Here's how the part is built. I have some questions about the finished solid (model axes, mm). A direction names the side the tool comes from. Coordinates: 2 decimals unless noted, no trailing zeros. Use CSV: the item, a comma, the result in double quotes. Start each with the question number.
```python
from build123d import *

# Parameters (mm, degrees)
ARM_DEPTH            = 2.54
LIGHTING_HOLES_REACH = 407.324
SKETCH3_R            = 10.563906398
SKETCH3_R_2          = 12.998589321
SKETCH3_R_3          = 14.959386689
SKETCH3_R_4          = 18.989420404
SKETCH3_R_5          = 20.414251761
SKETCH3_R_6          = 9.810598177
PIVOT_HOLES_REACH    = 407.324
SKETCH4_R            = 6.35
SKETCH5_R            = 2.54
EDGE_HOLES_DEPTH     = 2.54


with BuildPart() as part:
    # Sketch2 → Arm (new body)
    with BuildSketch(Plane(origin=(0, 0, 0), x_dir=(1, 0, 0), z_dir=(0, 1, 0))):
        with BuildLine():
            Line((-196.324159543, 163.36805283), (-239.26276826, 99.105883584))
            Line((-239.26276826, 99.105883584), (-258.976154185, 0))
            Line((-258.976154185, 0), (-239.26276826, -99.105883584))
            Line((-239.26276826, -99.105883584), (-183.12379479, -183.12379479))
            Line((-183.12379479, -183.12379479), (-110.768588535, -231.469997952))
            ThreePointArc((-110.768588535, -231.469997952), (-104.473118761, -249.064657285), (-119.482679559, -260.19650625))
            Line((-119.482679559, -260.19650625), (-231.805977786, -260.19650625))
            ThreePointArc((-231.805977786, -260.19650625), (-238.01719804, -258.573994365), (-242.641366534, -254.121032698))
            Line((-242.641366534, -254.121032698), (-263.949339301, -219.268704737))
            Line((-263.949339301, -219.268704737), (-305.536674142, -121.363782023))
            Line((-305.536674142, -121.363782023), (-310.771385022, 0))
            Line((-310.771385022, 0), (-287.766347466, 115.654133822))
            ThreePointArc((-287.766347466, 115.654133822), (-286.898137133, 118.373962558), (-285.444305631, 120.831121792))
            Line((-285.444305631, 120.831121792), (-238.69541851, 182.721728369))
            ThreePointArc((-238.69541851, 182.721728369), (-234.221705245, 186.435995307), (-228.561487284, 187.76709331))
            Line((-228.561487284, 187.76709331), (-209.365718386, 187.76709331))
            ThreePointArc((-209.365718386, 187.76709331), (-195.532827931, 179.475977845), (-196.324159543, 163.36805283))
        make_face()
    extrude(amount=ARM_DEPTH)

    # Sketch3 → Lighting Holes (cut, up to next)
    with BuildSketch(Plane(origin=(0, 2.54, 0), x_dir=(1, 0, 0), z_dir=(0, 1, 0)), mode=Mode.PRIVATE) as lighting_holes_sk1:
        with Locations(Location((-262.564493281, 112.317651632, 0), (0, 0, 270))):
            Circle(SKETCH3_R)
    lighting_holes_tool1 = extrude(lighting_holes_sk1.sketch, amount=-LIGHTING_HOLES_REACH, mode=Mode.PRIVATE) & part.part
    # Sketch3 → Lighting Holes (cut, up to next)
    with BuildSketch(Plane(origin=(0, 2.54, 0), x_dir=(1, 0, 0), z_dir=(0, 1, 0)), mode=Mode.PRIVATE) as lighting_holes_sk2:
        with Locations(Location((-273.830034517, 62.17947414, 0), (0, 0, 270))):
            Circle(SKETCH3_R_2)
    lighting_holes_tool2 = extrude(lighting_holes_sk2.sketch, amount=-LIGHTING_HOLES_REACH, mode=Mode.PRIVATE) & part.part
    # Sketch3 → Lighting Holes (cut, up to next)
    with BuildSketch(Plane(origin=(0, 2.54, 0), x_dir=(1, 0, 0), z_dir=(0, 1, 0)), mode=Mode.PRIVATE) as lighting_holes_sk3:
        with Locations(Location((-283.210721504, 0, 0), (0, 0, 270))):
            Circle(SKETCH3_R_3)
    lighting_holes_tool3 = extrude(lighting_holes_sk3.sketch, amount=-LIGHTING_HOLES_REACH, mode=Mode.PRIVATE) & part.part
    # Sketch3 → Lighting Holes (cut, up to next)
    with BuildSketch(Plane(origin=(0, 2.54, 0), x_dir=(1, 0, 0), z_dir=(0, 1, 0)), mode=Mode.PRIVATE) as lighting_holes_sk4:
        with Locations(Location((-275.563082601, -58.328881999, 0), (0, 0, 270))):
            Circle(SKETCH3_R_4)
    lighting_holes_tool4 = extrude(lighting_holes_sk4.sketch, amount=-LIGHTING_HOLES_REACH, mode=Mode.PRIVATE) & part.part
    # Sketch3 → Lighting Holes (cut, up to next)
    with BuildSketch(Plane(origin=(0, 2.54, 0), x_dir=(1, 0, 0), z_dir=(0, 1, 0)), mode=Mode.PRIVATE) as lighting_holes_sk5:
        with Locations(Location((-268.251334815, -119.393093751, 0), (0, 0, 270))):
            Circle(SKETCH3_R_5)
    lighting_holes_tool5 = extrude(lighting_holes_sk5.sketch, amount=-LIGHTING_HOLES_REACH, mode=Mode.PRIVATE) & part.part
    # Sketch3 → Lighting Holes (cut, up to next)
    with BuildSketch(Plane(origin=(0, 2.54, 0), x_dir=(1, 0, 0), z_dir=(0, 1, 0)), mode=Mode.PRIVATE) as lighting_holes_sk6:
        with Locations(Location((-229.533929598, 151.758024286, 0), (0, 0, 270))):
            Circle(SKETCH3_R_6)
    lighting_holes_tool6 = extrude(lighting_holes_sk6.sketch, amount=-LIGHTING_HOLES_REACH, mode=Mode.PRIVATE) & part.part
    add(lighting_holes_tool1.solids().sort_by_distance((-262.564493, 2.54, -112.317652))[0], mode=Mode.SUBTRACT)
    add(lighting_holes_tool2.solids().sort_by_distance((-273.830035, 2.54, -62.179474))[0], mode=Mode.SUBTRACT)
    add(lighting_holes_tool3.solids().sort_by_distance((-283.210722, 2.54, 0))[0], mode=Mode.SUBTRACT)
    add(lighting_holes_tool4.solids().sort_by_distance((-275.563083, 2.54, 58.328882))[0], mode=Mode.SUBTRACT)
    add(lighting_holes_tool5.solids().sort_by_distance((-268.251335, 2.54, 119.393094))[0], mode=Mode.SUBTRACT)
    add(lighting_holes_tool6.solids().sort_by_distance((-229.53393, 2.54, -151.758024))[0], mode=Mode.SUBTRACT)

    # Sketch4 → Pivot Holes (cut, up to next)
    with BuildSketch(Plane(origin=(0, 2.54, 0), x_dir=(1, 0, 0), z_dir=(0, 1, 0)), mode=Mode.PRIVATE) as pivot_holes_sk1:
        with Locations(Location((-119.482679559, -244.511556794, 0), (0, 0, 270))):
            Circle(SKETCH4_R)
    pivot_holes_tool1 = extrude(pivot_holes_sk1.sketch, amount=-PIVOT_HOLES_REACH, mode=Mode.PRIVATE) & part.part
    # Sketch4 → Pivot Holes (cut, up to next)
    with BuildSketch(Plane(origin=(0, 2.54, 0), x_dir=(1, 0, 0), z_dir=(0, 1, 0)), mode=Mode.PRIVATE) as pivot_holes_sk2:
        with Locations(Location((-227.432679559, -244.511556794, 0), (0, 0, 270))):
            Circle(SKETCH4_R)
    pivot_holes_tool2 = extrude(pivot_holes_sk2.sketch, amount=-PIVOT_HOLES_REACH, mode=Mode.PRIVATE) & part.part
    add(pivot_holes_tool1.solids().sort_by_distance((-119.48268, 2.54, 244.511557))[0], mode=Mode.SUBTRACT)
    add(pivot_holes_tool2.solids().sort_by_distance((-227.43268, 2.54, 244.511557))[0], mode=Mode.SUBTRACT)

    # Sketch5 → Edge Holes (cut)
    with BuildSketch(Plane(origin=(0, 2.54, 0), x_dir=(1, 0, 0), z_dir=(0, 1, 0))):
        with Locations(Location((-186.786270686, -186.786270686, 0), (0, 0, 270))):
            Circle(SKETCH5_R)
        with Locations(Location((-200.897754604, -165.666942533, 0), (0, 0, 270))):
            Circle(SKETCH5_R)
        with Locations(Location((-215.009238523, -144.547614381, 0), (0, 0, 270))):
            Circle(SKETCH5_R)
        with Locations(Location((-229.120722442, -123.428286228, 0), (0, 0, 270))):
            Circle(SKETCH5_R)
        with Locations(Location((-244.048023625, -101.088001256, 0), (0, 0, 270))):
            Circle(SKETCH5_R)
        with Locations(Location((-249.003317804, -76.176055134, 0), (0, 0, 270))):
            Circle(SKETCH5_R)
        with Locations(Location((-253.958611984, -51.264109011, 0), (0, 0, 270))):
            Circle(SKETCH5_R)
        with Locations(Location((-258.913906163, -26.352162889, 0), (0, 0, 270))):
            Circle(SKETCH5_R)
        with Locations(Location((-264.155677269, 0, 0), (0, 0, 270))):
            Circle(SKETCH5_R)
        with Locations(Location((-259.200383089, 24.911946122, 0), (0, 0, 270))):
            Circle(SKETCH5_R)
        with Locations(Location((-254.24508891, 49.823892244, 0), (0, 0, 270))):
            Circle(SKETCH5_R)
        with Locations(Location((-249.289794731, 74.735838367, 0), (0, 0, 270))):
            Circle(SKETCH5_R)
        with Locations(Location((-244.048023625, 101.088001256, 0), (0, 0, 270))):
            Circle(SKETCH5_R)
        with Locations(Location((-229.936539706, 122.207329408, 0), (0, 0, 270))):
            Circle(SKETCH5_R)
        with Locations(Location((-215.825055788, 143.326657561, 0), (0, 0, 270))):
            Circle(SKETCH5_R)
        with Locations(Location((-200.548025174, 166.190349614, 0), (0, 0, 270))):
            Circle(SKETCH5_R)
        with Locations(Location((-209.365718386, 182.68709331, 0), (0, 0, 270))):
            Circle(SKETCH5_R)
        with Locations(Location((-249.95111614, 159.392011893, 0), (0, 0, 270))):
            Circle(SKETCH5_R)
        with Locations(Location((-234.64184602, 179.659874346, 0), (0, 0, 270))):
            Circle(SKETCH5_R)
        with Locations(Location((-265.26038626, 139.12414944, 0), (0, 0, 270))):
            Circle(SKETCH5_R)
        with Locations(Location((-282.783958242, 114.663074986, 0), (0, 0, 270))):
            Circle(SKETCH5_R)
        with Locations(Location((-287.739252421, 89.751128864, 0), (0, 0, 270))):
            Circle(SKETCH5_R)
        with Locations(Location((-292.6945466, 64.839182741, 0), (0, 0, 270))):
            Circle(SKETCH5_R)
        with Locations(Location((-297.649840779, 39.927236619, 0), (0, 0, 270))):
            Circle(SKETCH5_R)
        with Locations(Location((-302.605134959, 15.015290497, 0), (0, 0, 270))):
            Circle(SKETCH5_R)
        with Locations(Location((-305.66976845, -0.391662485, 0), (0, 0, 270))):
            Circle(SKETCH5_R)
        with Locations(Location((-304.57522323, -25.768068274, 0), (0, 0, 270))):
            Circle(SKETCH5_R)
        with Locations(Location((-303.480678011, -51.144474063, 0), (0, 0, 270))):
            Circle(SKETCH5_R)
        with Locations(Location((-302.386132791, -76.520879852, 0), (0, 0, 270))):
            Circle(SKETCH5_R)
        with Locations(Location((-301.291587571, -101.89728564, 0), (0, 0, 270))):
            Circle(SKETCH5_R)
        with Locations(Location((-300.501066349, -120.225068676, 0), (0, 0, 270))):
            Circle(SKETCH5_R)
        with Locations(Location((-290.570595895, -143.603386762, 0), (0, 0, 270))):
            Circle(SKETCH5_R)
        with Locations(Location((-280.640125441, -166.981704849, 0), (0, 0, 270))):
            Circle(SKETCH5_R)
        with Locations(Location((-270.709654987, -190.360022936, 0), (0, 0, 270))):
            Circle(SKETCH5_R)
        with Locations(Location((-259.419983104, -216.93817365, 0), (0, 0, 270))):
            Circle(SKETCH5_R)
        with Locations(Location((-238.307211035, -251.471222119, 0), (0, 0, 270))):
            Circle(SKETCH5_R)
        with Locations(Location((-206.405977786, -255.11650625, 0), (0, 0, 270))):
            Circle(SKETCH5_R)
        with Locations(Location((-181.005977786, -255.11650625, 0), (0, 0, 270))):
            Circle(SKETCH5_R)
        with Locations(Location((-155.605977786, -255.11650625, 0), (0, 0, 270))):
            Circle(SKETCH5_R)
        with Locations(Location((-130.205977786, -255.11650625, 0), (0, 0, 270))):
            Circle(SKETCH5_R)
        with Locations(Location((-165.666942533, -200.897754604, 0), (0, 0, 270))):
            Circle(SKETCH5_R)
        with Locations(Location((-144.547614381, -215.009238523, 0), (0, 0, 270))):
            Circle(SKETCH5_R)
        with Locations(Location((-123.428286228, -229.120722442, 0), (0, 0, 270))):
            Circle(SKETCH5_R)
    extrude(amount=-EDGE_HOLES_DEPTH, mode=Mode.SUBTRACT)


solid = part.part
```
Item 1: Which directions (+Z, -Z, +X, -X, +Y, -Y) give clear straight access to the entire face, cutting with the end or side of a thin tool? Please do faces 1 (the flat face through (-262.4, 1.25, -151.34)), 2 (the flat face through (-217.49, 1.25, -131.69)).
Item 2: I want a section at A-A on y = 1.1. Count the separate pieces of the cut face and the enclosed holes in it, then the cut area to 3 significant figures.
Item 3: If I drill on line 1 along Z through (x, y) = (-221, 0.85); line 2 along X through (y, z) = (2.15, 25); line 3 along X through (y, z) = (1.95, -67), over which ranges is the centre line in solid material (lowest first)?
Item 4: I'm going to push a flat-ended pin straight in: pin 1 (4.5 mm diameter, centred on x = -238.31, z = 251.47, fed in from -Y). Where does the tip first touch, or does it pass through?
Item 5: Thinking about a two-plate mould opening in X: for faces 3 (the cylindrical face through (-231.297, 1.288, 239.472)), 4 (the cylindrical face through (-268.38, 1.29, -1.95)), 5 (the flat face through (-245, 2.54, 85)), 6 (the flat face through (-249.257, 1.252, 48.859)), which applies, +X half, -X half, draft (parallel to the pull), parting line (faces both ways), or undercut?
Geometry says:
1,face 1,"-Z, -X, +Y, -Y"
1,face 2,"+X, +Y, -Y"
2,separate pieces,"1"
2,enclosed holes,"51"
2,area,"27,500 mm2"
3,line 1,"-187.77 to -156.6, -146.92 to -126.44, 126.44 to 260.2"
3,line 2,"-309.69 to -307, -302.15 to -261.06, -256.76 to -254"
3,line 3,"-297.44 to -294.03, -291.36 to -285.9, -261.76 to -245.65"
4,pin 1,"through"
5,face 3,"undercut"
5,face 4,"undercut"
5,face 5,"draft"
5,face 6,"+X half"
